Part model, mm, in its own coordinate system. Face numbers are marked on the shaded views. Round coordinates to 2 decimals unless told otherwise and drop trailing zeros. Order: outer loops, then holes, each group sorted by start corner. A loop starts at its lowest first (then second) coordinate and runs counter-clockwise, first axis right, second up. Notation, with made-up numbers: M 61.5,72 L 120.5,72 A31 ccw 120.5,111 Z; hole C -11.75,79.5 d4. An arc over 180 degrees is marked long. Write each question's results on one line, items separated by ' | '. Start each with the question number.
1. Band-saw the part on B-B, the plane x = 0. List the corners of the cut face in (y, z).
2. Probe L1, parallel to X at y = 8.25, z = 0; L2, parallel to Z at x = -0.75, y = 7; L3, parallel to X at y = 4.25, z = 1.25. List the from-to ranges inside material, lowest first. Write a range as [from, to].
3. Band-saw the part on C-C, the plane y = 8.75. List the corners of the cut face in (x, z), then the cut area to 3 significant figures.
4. Two-plate mould, pull along Z, no slides. Class the marked faces 1, 2 and 3: +Z half, -Z half, draft (parallel to the pull), parting line (faces both ways), or undercut.
5. Drop flat-ended pins along their axis: pin 1 Ø1.5 at (x, z) = (0.5, -4) entering from -Y; pin 2 Ø6 at (y, z) = (2.5, 3) entering from +X; pin 3 Ø1.5 at (x, y) = (-3, 4.5) entering from +Z; pin 4 Ø6 at (y, z) = (6, -4) entering from +X. Give the stop position or say it passes through.
6. Band-saw the part on D-D, the plane y = 2.75. List the corners of the cut face in (x, z).
7. Band-saw the part on A-A, the plane z = 0. List the corners of the cut face in (x, y).
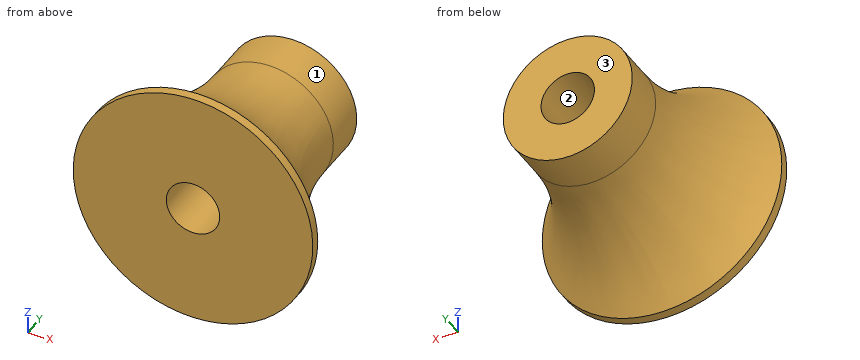
```python
from build123d import *

# Parameters (mm, degrees)
SKETCH1_R           = 3.5
SKETCH1_R_2         = 1.45
BOSS_EXTRUDE1_DEPTH = 10
SKETCH2_R           = 6.5
SKETCH2_R_2         = 3.5
SKETCH2_R_3         = 1.45
BOSS_EXTRUDE2_DEPTH = 0.5
FILLET1_R           = 10


with BuildPart() as part:
    # Sketch1 → Boss-Extrude1 (new body)
    with BuildSketch(Plane(origin=(0, 0, 0), x_dir=(1, 0, 0), z_dir=(0, 1, 0))):
        with Locations(Location((0, 0, 0), (0, 0, 270))):
            Circle(SKETCH1_R)
        with Locations(Location((0, 0, 0), (0, 0, 270))):
            Circle(SKETCH1_R_2, mode=Mode.SUBTRACT)
    extrude(amount=BOSS_EXTRUDE1_DEPTH)

    # Sketch2 → Boss-Extrude2 (add)
    # profile 1 of 2: a face of its own
    with BuildSketch(Plane.XZ):
        with Locations(Location((0, 0, 0), (0, 0, 270))):
            Circle(SKETCH2_R)
        with Locations(Location((0, 0, 0), (0, 0, 270))):
            Circle(SKETCH2_R_2, mode=Mode.SUBTRACT)
    # profile 2 of 2: a face of its own
    with BuildSketch(Plane.XZ):
        with Locations(Location((0, 0, 0), (0, 0, 270))):
            Circle(SKETCH2_R_2)
        with Locations(Location((0, 0, 0), (0, 0, 90))):
            Circle(SKETCH2_R_3, mode=Mode.SUBTRACT)
    extrude(amount=-BOSS_EXTRUDE2_DEPTH)

    # Fillet1
    # the kernel refuses this fillet: 10 mm, written as the material it adds along each edge
    with BuildSketch(Plane(origin=(0, 0.5, 0), x_dir=(0, 0, 1), z_dir=(1, 0, 0))) as fillet1_piece_1:
        with BuildLine():
            CenterArc((13.5, -7.141428429), FILLET1_R, 134.427004001, 45.572995999)
            Line((3.5, -7.141428429), (3.3, -7.141428429))
            Line((3.3, -7.141428429), (3.3, 0))
            Line((3.3, 0), (3.5, 0.2))
            ThreePointArc((3.5, 0.2), (5, 0.2), (6.36, 0.142828569))
            Line((6.36, 0.142828569), (6.5, 0))
        make_face()
    revolve(axis=Axis((0, 0.5, 0), (0, -1, 0)))


solid = part.part
```
Solution:
1) outline: M 0,-6.5 L 0.5,-6.5 A10 cw 7.64,-3.5 L 10,-3.5 L 10,-1.45 L 0,-1.45 Z; M 0,1.45 L 10,1.45 L 10,3.5 L 7.64,3.5 A10 cw 0.5,6.5 L 0,6.5 Z
2) L1: [-3.5, -1.45], [1.45, 3.5] | L2: [-3.44, -1.24], [1.24, 3.44] | L3: [-3.9, -0.73], [0.73, 3.9]
3) outline: C 0,0 d7; hole C 0,0 d2.9 | area: 31.9 mm^2
4) face 1: parting line | face 2: undercut | face 3: draft
5) pin 1: y = 0 | pin 2: x = 6.45 | pin 3: z = 3.41 | pin 4: x = 3.8
6) outline: C 0,0 d9.56; hole C 0,0 d2.9
7) outline: M -6.5,0 L -1.45,0 L -1.45,10 L -3.5,10 L -3.5,7.64 A10 cw -6.5,0.5 Z; M 1.45,0 L 6.5,0 L 6.5,0.5 A10 cw 3.5,7.64 L 3.5,10 L 1.45,10 Z
